Geometry check sheet. Reference: the model listing, model coordinates, mm. A direction names the side the tool comes from. Round coordinates to 2 decimals unless told otherwise and drop trailing zeros. Write each loop counter-clockwise with the first axis right and the second up, starting at its lowest first coordinate (ties: lowest second). Pieces come first, ordered by that corner, then holes.
Item 1: Cross-section at B-B (x = -12.5). Enter the section's corners in (y, z) (3 decimals), then the cut area to 3 significant figures.
Item 2: Draft check along Z on faces 1 (the face through (-24.74, -26.327, 10.916)), 2 (the face through (5, 24, 0)), 3 (the face through (0.357, 14.122, -0.29)). Enter one of: pulls with the +Z half, pulls with the -Z half, needs draft (parallel to the pull), parting line crosses it, or undercut.
Item 3: Access from +Z, -Z, +X, -X, +Y, -Y to the whole of each face (thin tool, end or side, straight path). Record for faces 4 (the face through (3.018, 2.994, -22.804)), 5 (the face through (-25.674, 14.169, 0.291)), 6 (the face through (25.674, -14.169, 0.291)).
Item 4: Scan lines: probe 1 along Z at (x, y) = (7, -1); probe 2 along X at (y, z) = (-10, 23); probe 3 along Y at (x, z) = (-3, 10). Record each from-to range of solid material in increasing order.
Item 5: Cross-section at A-A (x = 13). Enter the section's corners in (y, z) (3 decimals).
Item 6: Depth check by flat-ended pin: P1, Ø0.5, axis at x = -11, z = -14, coming from the +Y side; P2, Ø3.5, axis at x = 8.5, y = -0.5, coming from the +Z side; P3, Ø1, axis at x = 9.5, y = -3, coming from the -Z side. Enter the tip coordinate at first touch or a pass-through.
Autodesk Inventor part; units mm, degrees
ref_plane "YZ Plane" through (0, 0, 0) normal (1, 0, 0) x (0, 1, 0)
ref_plane "XZ Plane" through (0, 0, 0) normal (0, 1, 0) x (-1, 0, 0)
ref_plane "XY Plane" through (0, 0, 0) normal (0, 0, 1) x (1, 0, 0)
sketch "Эскиз1" plane through (0, 0, 0) normal (0, 0, 1) x (1, 0, 0)
  line L0 (-26.5, 0) -> (26.5, 0)
  line L1 (-26.5, -14.3929) -> (-26.5, -27.5)
  line L2 (-25.5, -28.5) -> (-24, -28.5)
  line L3 (-26.5, -14.3929) -> (-25.5, -14.125)
  line L4 (-25.5, -14.125) -> (25.5, -14.125)
  line L5 (-25.5, -28.5) -> (-26.5, -27.5)
  line L6 (-21, -31.5) -> (-21, -36.75)
  arc A0 (-21, -31.5) -> (-24, -28.5) centre (-24, -31.5) ccw
  line L7 (-21, -36.75) -> (-0.5, -36.75)
  line L8 (-0.5, -36.75) -> (-0.5, -30.5)
  line L9 (-0.5, -30.5) -> (1, -29)
  line L10 (1, -29) -> (1, -23)
  line L11 (1, -23) -> (5, -23)
  line L12 (5, -23) -> (5, -29)
  line L13 (5, -29) -> (6.5, -30.5)
  line L14 (6.5, -30.5) -> (6.5, -45.125)
  line L15 (6.5, -45.125) -> (26.5, -45.125)
  line L16 (26.5, -45.125) -> (26.5, -14.3929)
  line L17 (26.5, -14.3929) -> (25.5, -14.125)
  point P0 (0, 0)
  point P1 (0, 0)
  point P2 (-26.5, -28.5)
  dimension "d0" = 53
  dimension "d1" = 28.25
  dimension "d2" = 15
  dimension "d3" = 57
  dimension "d4" = 1
  dimension "d5" = 1
  dimension "d6" = 45
  dimension "d7" = 3
  dimension "d8" = 73.5
  dimension "d9" = 5.5
  dimension "d10" = 7
  dimension "d11" = 4
  dimension "d12" = 46
  dimension "d13" = 21.5
  dimension "d14" = 20
  dimension "d15" = 58
  dimension "d16" = 45
  dimension "d17" = 15
  dimension "d18" = 1
  dimension "d19" = 90.25
revolve "Вращение1" add sketch "Эскиз1" angle 360 about axis through (-26.5, 0, 0) along (1, 0, 0)
sketch "Эскиз2" plane through (0, 0, 0) normal (0, 0, 1) x (1, 0, 0)
  line L0 (26.5, 45.125) -> (6.5, 45.125)
  line L1 (26.5, 0) -> (6.5, 0)
  line L2 (26.5, 45.125) -> (26.5, -45.125)
  line L3 (6.5, 45.125) -> (26.5, 45.125)
  line L4 (26.5, 45.125) -> (26.5, 31.5)
  line L5 (26.5, 31.5) -> (6.5, 31.5)
  line L6 (6.5, 31.5) -> (6.5, 45.125)
  point P0 (0, 0)
  dimension "d21" = 63
revolve "Вращение2" cut sketch "Эскиз2" angle 360 about axis through (26.5, 0, 0) along (-1, 0, 0)
fillet "Сопряжение1" radius 0.75 2 edges at (1, 23, 0) (5, 23, 0)
sketch "Эскиз3" plane through (0, 0, 0) normal (0, 0, 1) x (1, 0, 0)
  line L0 (-21, 36.75) -> (-21, -36.75)
  line L1 (-0.5, 36.75) -> (-0.5, -36.75)
  line L2 (-21, 31.5) -> (-21, -31.5)
  line L3 (-21, 0) -> (0, 0)
  line L4 (-21, 36.75) -> (-0.5, 36.75)
  line L5 (-0.5, 36.75) -> (-0.5, 30)
  line L6 (-0.5, 30) -> (-21, 30)
  line L7 (-21, 30) -> (-21, 36.75)
  point P0 (-21, 30)
  dimension "d24" = 60
revolve "Вращение3" cut sketch "Эскиз3" angle 360 about axis through (-21, 0, 0) along (1, 0, 0) contours L4 L1 L6 L0
sketch "Эскиз4" plane through (-26.5, 0, 0) normal (-1, 0, 0) x (0, 0, 1)
  line L0 (-14.5451, 1.5) -> (-14.0451, 1.5)
  line L1 (-14.0451, 1.5) -> (-14.0451, -1.5)
  line L2 (-14.0451, -1.5) -> (-14.5451, -1.5)
  line L3 (-14.5451, -1.5) -> (-14.5451, 1.5)
  circle A0 centre (0, 0) radius 14.125
  point P0 (0, 0)
  point P1 (-14.0451, 0)
  dimension "d26" = 3
  dimension "d27" = 0.5
extrude "Выдавливание1" cut sketch "Эскиз4" against normal through all contours L0 A0 L2 L3 | L1 A0 picked at (-14.0688, 0.1669)
mirror "Зеркальное отражение1" about plane through (0, 0, 0) normal (0, 0, 1) of "Выдавливание1"
properties part number "71. Блок шестерен заднего хода"
Resolved:
1. outline: circle Ø60 at (0, 0); hole (-1.5, -14.545) - (1.5, -14.545) - (1.5, -14.045) arc R14.125 ccw to (1.5, 14.045) - (1.5, 14.545) - (-1.5, 14.545) - (-1.5, 14.045) arc R14.125 ccw to (-1.5, -14.045) - close
1. area: 2,200 mm2
2. face 1: parting line crosses it
2. face 2: needs draft
2. face 3: undercut
3. face 4: none
3. face 5: -X
3. face 6: +X
4. probe 1: z = -31.48 to -14.55, 14.55 to 31.48
4. probe 2: x = -26.5 to 1, 5 to 26.5
4. probe 3: y = -28.28 to -9.98, 9.98 to 28.28
5. outline: circle Ø63 at (0, 0); hole (-1.5, -14.545) - (1.5, -14.545) - (1.5, -14.045) arc R14.125 ccw to (1.5, 14.045) - (1.5, 14.545) - (-1.5, 14.545) - (-1.5, 14.045) arc R14.125 ccw to (-1.5, -14.045) - close
6. P1: stops at y = 26.66
6. P2: stops at z = 31.5
6. P3: stops at z = -31.4
